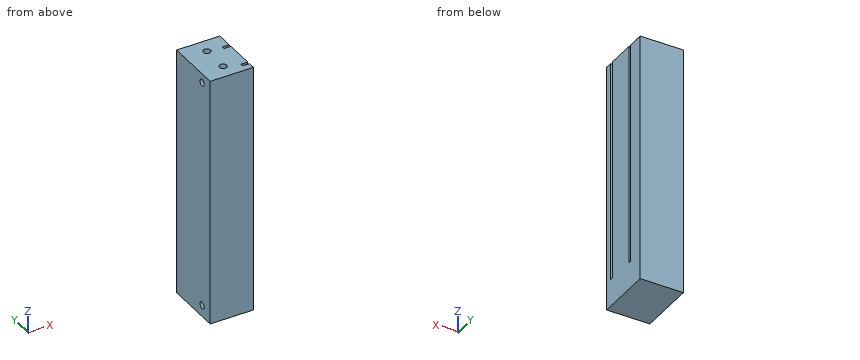
```python
from build123d import *

# Parameters (mm, degrees)
SKETCH1_W                    = 19
SKETCH1_H                    = 110
BLOCK_DEPTH                  = 25
SKETCH2_W                    = 98
SKETCH2_H                    = 1.25
SLIDES_DEPTH                 = 3
SKETCH3_R                    = 1.5
MOUNTING_HOLES_DEPTH         = 10
SKETCH5_R                    = 1.575
CUT_EXTRUDE1_DEPTH           = 15
CUT_EXTRUDE1_DRAFT           = -1
CUT_EXTRUDE1_PROFILE_2_DEPTH = 15
CUT_EXTRUDE1_PROFILE_2_DRAFT = -1


with BuildPart() as part:
    # Sketch1 → Block (new body)
    with BuildSketch(Plane(origin=(0, 0, 0), x_dir=(1, 0, 0), z_dir=(0, 1, 0))):
        Rectangle(SKETCH1_W, SKETCH1_H)
    extrude(amount=BLOCK_DEPTH)

    # Sketch2 → Slides (cut)
    with BuildSketch(Plane(origin=(9.5, 0, 0), x_dir=(0, 0, -1), z_dir=(1, 0, 0))):
        with Locations((-6, 3.625)):
            Rectangle(SKETCH2_W, SKETCH2_H)
        with Locations((-6, 17.375)):
            Rectangle(SKETCH2_W, SKETCH2_H)
    extrude(amount=-SLIDES_DEPTH, mode=Mode.SUBTRACT)

    # Sketch3 → Mounting Holes (cut)
    with BuildSketch(Plane.ZY.offset(9.5)):
        with Locations((-50, 6)):
            Circle(SKETCH3_R)
        with Locations((51, 6)):
            Circle(SKETCH3_R)
    extrude(amount=-MOUNTING_HOLES_DEPTH, mode=Mode.SUBTRACT)


with BuildPart() as cut_extrude1_tool:
    # Sketch5 → Cut-Extrude1 (with draft: the straight prism first)
    with BuildSketch(Plane.XY.offset(55)):
        with Locations((0, 18.5)):
            Circle(SKETCH5_R)
    extrude(amount=-CUT_EXTRUDE1_DEPTH)
    # Cut-Extrude1: the draft: its side faces are tilted about the plane it starts from
    cut_extrude1_sides = [cut_extrude1_tool.faces().sort_by_distance(p)[0] for p in [
        (-1.575, 18.5, 47.5),
    ]]
    draft(cut_extrude1_sides, Plane.XY.offset(55), CUT_EXTRUDE1_DRAFT)


with BuildPart() as part_1:
    add(part.part)

    # Cut-Extrude1: cut by cut_extrude1_tool
    add(cut_extrude1_tool.part, mode=Mode.SUBTRACT)


with BuildPart() as cut_extrude1_profile_2_tool:
    # Sketch5 → Cut-Extrude1 profile 2 (with draft: the straight prism first)
    with BuildSketch(Plane.XY.offset(55)):
        with Locations((0, 6.5)):
            Circle(SKETCH5_R)
    extrude(amount=-CUT_EXTRUDE1_PROFILE_2_DEPTH)
    # Cut-Extrude1 profile 2: the draft: its side faces are tilted about the plane it starts from
    cut_extrude1_profile_2_sides = [cut_extrude1_profile_2_tool.faces().sort_by_distance(p)[0] for p in [
        (-1.575, 6.5, 47.5),
    ]]
    draft(cut_extrude1_profile_2_sides, Plane.XY.offset(55), CUT_EXTRUDE1_PROFILE_2_DRAFT)


with BuildPart() as part_2:
    add(part_1.part)

    # Cut-Extrude1 profile 2: cut by cut_extrude1_profile_2_tool
    add(cut_extrude1_profile_2_tool.part, mode=Mode.SUBTRACT)


solid = part_2.part
```
Geometry check sheet. Reference: the model listing, model coordinates, mm. Give positions to 0.01 mm unless a question says otherwise; leave off trailing zeros. Loops run counter-clockwise (first coordinate to the right, second up) from the corner with the lowest first, then second, coordinate; pieces in that order, holes last. Notation, with made-up numbers: M 73.5,38.5 L 101.5,38.5 A30 ccw 101.5,77.5 Z; hole C -9,21 d10. An arc over 180 degrees is marked long. Answer as CSV lines item,"result".
Item 1: Cross-section at B-B on z = -50. Record the cut outline in (x, y).
Values:
outline,"M -9.5,0 L 9.5,0 L 9.5,25 L -9.5,25 L -9.5,7.5 L 0.5,7.5 L 0.5,4.5 L -9.5,4.5 Z"
Item 2: Depth check by flat-ended pin: P1, Ø2.5, axis at x = 7.5, z = -13, coming from the -Y side; P2, Ø2, axis at x = 0, y = 6.5, coming from the +Z side; P3, Ø0.5, axis at y = 5, z = 51.5, coming from the -X side. Enter the tip coordinate at first touch or a pass-through.
Values:
P1,"stops at y = 0"
P2,"stops at z = 40"
P3,"stops at x = 0.5"
Item 3: Material ranges on line 1 (Y direction, x = 7, z = -14); line 2 (Y direction, x = -3.25, z = 51); line 3 (X direction, y = 17.5, z = 20.5), recorded low to high.
Values:
line 1,"y = 0 to 3, 4.25 to 16.75, 18 to 25"
line 2,"y = 0 to 4.5, 7.5 to 25"
line 3,"x = -9.5 to 6.5"
Item 4: Cross-section at A-A on z = -26.5. Record the cut outline in (x, y).
Values:
outline,"M -9.5,0 L 9.5,0 L 9.5,3 L 6.5,3 L 6.5,4.25 L 9.5,4.25 L 9.5,16.75 L 6.5,16.75 L 6.5,18 L 9.5,18 L 9.5,25 L -9.5,25 Z"
